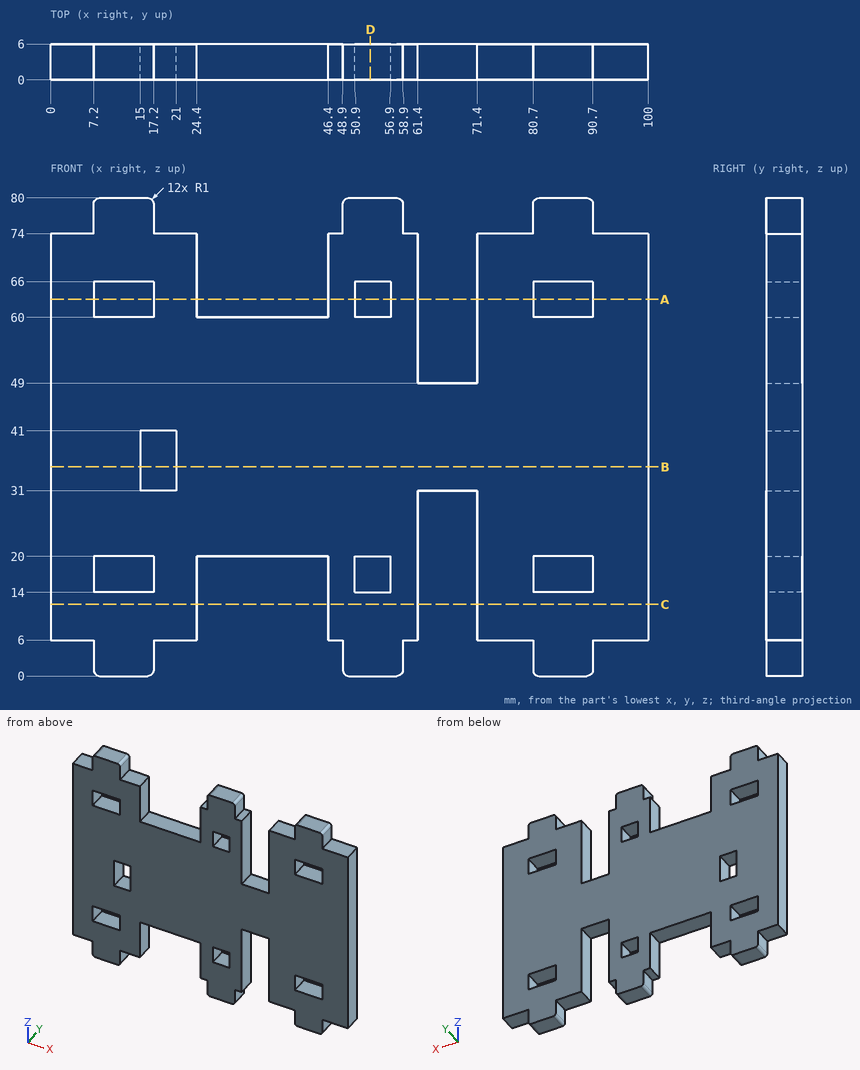
Job drawing, mm, ordinate dimensions from the low corner. One solid piece. Coordinates: 2 decimals unless noted, no trailing zeros. Write each loop counter-clockwise with the first axis right and the second up, starting at its lowest first coordinate (ties: lowest second). Pieces come first, ordered by that corner, then holes. Notation, with made-up numbers: (83, 38) - (130, 38) arc R23 ccw to (130, 67) - close; hole circle Ø4 at (42, -26). An arc over 180 degrees is marked (long way). Use a Markdown table: item, result. Add a question column.
Item 1: Band-saw the part on B-B, the plane z = 35. Give the cut face in (x, y), and give its area (3 significant figures).
Item 2: Drill centre lines: L1, parallel to X at y = 5, z = 75; L2, parallel to Z at x = 10, y = 3.95; L3, parallel to X at y = 1.65, z = 72. Where is each one in solid material? Low to high. Write a range as from..to.
Item 3: Band-saw the part on C-C, the plane z = 12. Give the cut face in (x, y).
Item 4: Band-saw the part on A-A, the plane z = 63. Give the cut face in (x, y), and give its area (3 significant figures).
Item 5: Band-saw the part on D-D, the plane x = 53.5. Give the cut face in (y, z).
Item 6: Flat gauge pins, fed straight in: pin 1 (2.5 mm diameter, centred on y = 2, z = 3.5, fed in from +X); pin 2 (1.8 mm diameter, centred on x = 33, y = 3.5, fed in from +Z); pin 3 (1 mm diameter, centred on x = 75, y = 5, fed in from -Z). Where does each tip first touch, or does it go through?
Numbers:
| question | item | result |
|---|---|---|
| 1 | outline | (0, 0) - (15, 0) - (15, 6) - (0, 6) - close; (21, 0) - (100, 0) - (100, 6) - (21, 6) - close |
| 1 | area | 564 mm2 |
| 2 | L1 | 7.2..17.2, 48.9..58.9, 80.7..90.7 |
| 2 | L2 | 0..14, 20..60, 66..80 |
| 2 | L3 | 0..24.4, 46.4..61.4, 71.4..100 |
| 3 | outline | (0, 0) - (24.4, 0) - (24.4, 6) - (0, 6) - close; (46.4, 0) - (61.4, 0) - (61.4, 6) - (46.4, 6) - close; (71.4, 0) - (100, 0) - (100, 6) - (71.4, 6) - close |
| 4 | outline | (0, 0) - (7.2, 0) - (7.2, 6) - (0, 6) - close; (17.2, 0) - (24.4, 0) - (24.4, 6) - (17.2, 6) - close; (46.4, 0) - (50.9, 0) - (50.9, 6) - (46.4, 6) - close; (56.9, 0) - (61.4, 0) - (61.4, 6) - (56.9, 6) - close; (71.4, 0) - (80.7, 0) - (80.7, 6) - (71.4, 6) - close; (90.7, 0) - (100, 0) - (100, 6) - (90.7, 6) - close |
| 4 | area | 252 mm2 |
| 5 | outline | (0, 0) - (6, 0) - (6, 14) - (0, 14) - close; (0, 20) - (6, 20) - (6, 60) - (0, 60) - close; (0, 66) - (6, 66) - (6, 80) - (0, 80) - close |
| 6 | pin 1 | x = 90.7 |
| 6 | pin 2 | z = 60 |
| 6 | pin 3 | z = 6 |
